```python
from build123d import *
from build123d.topology import SkipClean

# Parameters (mm, degrees)
SKETCH_1_R               = 705
EXTRUDE_1_DEPTH          = 25
CUT_EXTRUDE_1_REACH      = 999.334
PATTERN_CIRCULAR_1_COUNT = 4
CUT_EXTRUDE_2_REACH      = 999.177
SKETCH_8_R               = 60
CUT_EXTRUDE_3_DEPTH      = 998.177266087
CUT_EXTRUDE_7_DEPTH      = 998.177266087
CUT_EXTRUDE_8_DEPTH      = 998.177266087
SKETCH_18_R              = 40
CUT_EXTRUDE_13_DEPTH     = 998.177266087
SKETCH_19_R              = 3
CUT_EXTRUDE_14_DEPTH     = 100
CUT_EXTRUDE_15_DEPTH     = 8


with BuildPart() as part:
    # 草图1 → 凸台-拉伸1 (new body)
    with BuildSketch(Plane(origin=(0, 0, 0), x_dir=(1, 0, 0), z_dir=(0, 1, 0))):
        with Locations(Location((0, 0, 0), (0, 0, 270))):
            Circle(SKETCH_1_R)
    extrude(amount=EXTRUDE_1_DEPTH)

    # 草图2 → 切除-拉伸1 (cut, up to next)
    with BuildSketch(Plane(origin=(0, 25, 0), x_dir=(1, 0, 0), z_dir=(0, 1, 0)), mode=Mode.PRIVATE) as cut_extrude_1_sk1:
        with BuildLine():
            Line((-12.5, -699.994189271), (-12.5, -704.889175687))
            ThreePointArc((-12.5, -704.889175687), (0, -705), (12.5, -704.889175687))
            Line((12.5, -704.889175687), (12.5, -699.994189271))
            Line((12.5, -699.994189271), (0, -678.343554177))
            Line((0, -678.343554177), (-12.5, -699.994189271))
        make_face()
    cut_extrude_1_tool1 = extrude(cut_extrude_1_sk1.sketch, amount=-CUT_EXTRUDE_1_REACH, mode=Mode.PRIVATE) & part.part
    cut_extrude_1 = cut_extrude_1_tool1.solids().sort_by_distance((0, 25, 695.82939))[0]
    add(cut_extrude_1, mode=Mode.SUBTRACT)

    # 阵列(圆周)1: 切除-拉伸1 ×4 about axis
    pattern_circular_1_axis = Axis((0, 0, 0), (0, 1, 0))
    for i in range(1, PATTERN_CIRCULAR_1_COUNT):
        add(cut_extrude_1.rotate(pattern_circular_1_axis, i * 360 / PATTERN_CIRCULAR_1_COUNT), mode=Mode.SUBTRACT)

    # 草图8 → 切除-拉伸2 (cut, up to next)
    with BuildSketch(Plane(origin=(0, 25, 0), x_dir=(1, 0, 0), z_dir=(0, 1, 0)), mode=Mode.PRIVATE) as cut_extrude_2_sk1:
        with Locations(Location((247.487373415, -247.487373415, 0), (0, 0, 270))):
            Circle(SKETCH_8_R)
    cut_extrude_2_tool1 = extrude(cut_extrude_2_sk1.sketch, amount=-CUT_EXTRUDE_2_REACH, mode=Mode.PRIVATE) & part.part
    # 草图8 → 切除-拉伸2 (cut, up to next)
    with BuildSketch(Plane(origin=(0, 25, 0), x_dir=(1, 0, 0), z_dir=(0, 1, 0)), mode=Mode.PRIVATE) as cut_extrude_2_sk2:
        with Locations(Location((-212.132034356, -212.132034356, 0), (0, 0, 270))):
            Circle(SKETCH_8_R)
    cut_extrude_2_tool2 = extrude(cut_extrude_2_sk2.sketch, amount=-CUT_EXTRUDE_2_REACH, mode=Mode.PRIVATE) & part.part
    # 草图8 → 切除-拉伸2 (cut, up to next)
    with BuildSketch(Plane(origin=(0, 25, 0), x_dir=(1, 0, 0), z_dir=(0, 1, 0)), mode=Mode.PRIVATE) as cut_extrude_2_sk3:
        with Locations(Location((-212.132034356, 212.132034356, 0), (0, 0, 270))):
            Circle(SKETCH_8_R)
    cut_extrude_2_tool3 = extrude(cut_extrude_2_sk3.sketch, amount=-CUT_EXTRUDE_2_REACH, mode=Mode.PRIVATE) & part.part
    # 草图8 → 切除-拉伸2 (cut, up to next)
    with BuildSketch(Plane(origin=(0, 25, 0), x_dir=(1, 0, 0), z_dir=(0, 1, 0)), mode=Mode.PRIVATE) as cut_extrude_2_sk4:
        with Locations(Location((212.132034356, 212.132034356, 0), (0, 0, 270))):
            Circle(SKETCH_8_R)
    cut_extrude_2_tool4 = extrude(cut_extrude_2_sk4.sketch, amount=-CUT_EXTRUDE_2_REACH, mode=Mode.PRIVATE) & part.part
    add(cut_extrude_2_tool1.solids().sort_by_distance((247.487373, 25, 247.487373))[0], mode=Mode.SUBTRACT)
    add(cut_extrude_2_tool2.solids().sort_by_distance((-212.132034, 25, 212.132034))[0], mode=Mode.SUBTRACT)
    add(cut_extrude_2_tool3.solids().sort_by_distance((-212.132034, 25, -212.132034))[0], mode=Mode.SUBTRACT)
    add(cut_extrude_2_tool4.solids().sort_by_distance((212.132034, 25, -212.132034))[0], mode=Mode.SUBTRACT)

    # 草图9 → 切除-拉伸3 (cut, through all)
    with BuildSketch(Plane(origin=(0, 25, 0), x_dir=(1, 0, 0), z_dir=(0, 1, 0))):
        Polygon((388.545974556, -190.514916099), (515.825974556, -63.236474876), (643.105974556, -190.514916099), (515.825974556, -317.793357321), align=None)
    extrude(amount=-CUT_EXTRUDE_3_DEPTH, mode=Mode.SUBTRACT)

    # 草图13 → 切除-拉伸7 (cut, through all)
    with BuildSketch(Plane.XZ):
        Polygon((165.039343844, 165.039343844), (398.093317994, -68.014630305), (332.597815836, -133.510132463), (99.543841687, 99.543841687), align=None)
    extrude(amount=-CUT_EXTRUDE_7_DEPTH, mode=Mode.SUBTRACT)

    # 草图14 → 切除-拉伸8 (cut, through all)
    with BuildSketch(Plane.XZ):
        Polygon((165.039343844, 165.039343844), (99.543841687, 99.543841687), (76.501917102, 122.585766271), (141.99741926, 188.081268429), align=None)
    extrude(amount=-CUT_EXTRUDE_8_DEPTH, mode=Mode.SUBTRACT)

    # 草图18 → 切除-拉伸13 (cut, through all)
    with BuildSketch(Plane(origin=(0, 25, 0), x_dir=(1, 0, 0), z_dir=(0, 1, 0))):
        with Locations(Location((-156.54417142, -331.667653242, 0), (0, 0, 270))):
            Circle(SKETCH_18_R)
    extrude(amount=-CUT_EXTRUDE_13_DEPTH, mode=Mode.SUBTRACT)

    # 草图19 → 切除-拉伸14 (cut)
    with BuildSketch(Plane.XZ):
        with Locations(Location((-10.777149233, 258.231573261, 0), (0, 0, 270))):
            Circle(SKETCH_19_R)
        with Locations(Location((-191.089378436, 438.543802464, 0), (0, 0, 270))):
            Circle(SKETCH_19_R)
        with Locations(Location((3.36498639, 272.373708885, 0), (0, 0, 90))):
            Circle(SKETCH_19_R)
        with Locations(Location((-176.947242812, 452.685938088, 0), (0, 0, 90))):
            Circle(SKETCH_19_R)
    extrude(amount=-CUT_EXTRUDE_14_DEPTH, mode=Mode.SUBTRACT)

    # 草图20 → 切除-拉伸15 (cut)
    with SkipClean():  # the faces are left unmerged after this step: merging them gives an invalid solid
        with BuildSketch(Plane(origin=(0, 25, 0), x_dir=(1, 0, 0), z_dir=(0, 1, 0))):
            with BuildLine():
                Line((169.705627485, 169.705627485), (84.852813742, 254.558441227))
                ThreePointArc((84.852813742, 254.558441227), (84.852813742, 339.41125497), (169.705627485, 339.41125497))
                Line((169.705627485, 339.41125497), (254.558441227, 254.558441227))
                ThreePointArc((254.558441227, 254.558441227), (254.558441227, 169.705627485), (169.705627485, 169.705627485))
            make_face()
            with BuildLine():
                Line((-169.705627485, -169.705627485), (-254.558441227, -84.852813742))
                ThreePointArc((-254.558441227, -84.852813742), (-339.41125497, -84.852813742), (-339.41125497, -169.705627485))
                Line((-339.41125497, -169.705627485), (-254.558441227, -254.558441227))
                ThreePointArc((-254.558441227, -254.558441227), (-169.705627485, -254.558441227), (-169.705627485, -169.705627485))
            make_face()
            with BuildLine():
                Line((-169.705627485, 169.705627485), (-254.558441227, 84.852813742))
                ThreePointArc((-254.558441227, 84.852813742), (-339.41125497, 84.852813742), (-339.41125497, 169.705627485))
                Line((-339.41125497, 169.705627485), (-254.558441227, 254.558441227))
                ThreePointArc((-254.558441227, 254.558441227), (-169.705627485, 254.558441227), (-169.705627485, 169.705627485))
            make_face()
            with BuildLine():
                Line((289.913780286, -289.913780286), (205.060966544, -374.766594029))
                ThreePointArc((205.060966544, -374.766594029), (120.208152802, -374.766594029), (120.208152802, -289.913780286))
                Line((120.208152802, -289.913780286), (205.060966544, -205.060966544))
                ThreePointArc((205.060966544, -205.060966544), (289.913780286, -205.060966544), (289.913780286, -289.913780286))
            make_face()
        extrude(amount=-CUT_EXTRUDE_15_DEPTH, mode=Mode.SUBTRACT)


solid = part.part
```
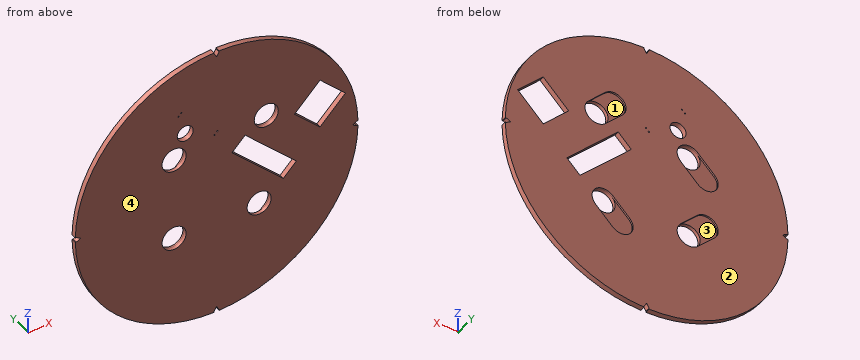
The listing builds one solid part. Answer for the finished solid, in the listing's coordinates (mm). Face numbers are marked on the shaded views. A direction names the side the tool comes from. Give positions to 0.01 mm unless a question says otherwise; leave off trailing zeros. Loops run counter-clockwise (first coordinate to the right, second up) from the corner with the lowest first, then second, coordinate; pieces in that order, holes last. Notation, with made-up numbers: (45, 39.5) - (88, 39.5) arc R3 cw to (88, 44.5) - close; hole circle Ø6 at (22.25, 25). An arc over 180 degrees is marked (long way). Return JSON: item names as keys, results as strings. Group by question number.
1. Find section C-C (y = 13.25). State how many separate pieces and enclosed holes the cut face has, then the cut area to 3 significant figures.
2. Determine the mould class of the marked faces 1 and 2 for opening direction X: pulls with the +X half, pulls with the -X half, needs draft (parallel to the pull), parting line crosses it, or undercut.
3. Find section A-A (x = 571.5). Write down the section's boundary in (y, z).
4. Find section B-B (z = -471). Write down the section's boundary in (x, y).
5. Which of the six approach directions +Z, -Z, +X, -X, +Y, -Y give full straight-line access (tool end or side, diameter ignored) to the marked faces 3 and 4?
6. Find section D-D (x = -490). Write down the section's boundary in (y, z).
7. Straight lines are drawn through the part: line 1 (Z direction, x = 257.5, y = 15.75); line 2 (Z direction, x = 234.5, y = 23.75); line 3 (X direction, y = 3, z = 144). For each, find the intervals that lie inside material, in ascending order. Write a range as [from, to].
8. Given pin 1 Ø3 at (x, y) = (427.5, 18.5) entering from +Z; pin 2 Ø12 at (y, z) = (10, 110.5) entering from -X; pin 3 Ø5 at (x, y) = (-358.5, 17.5) entering from -Z, each flat-ended and moving along its own axis, determine where each tip first touches the part or whether it passes through.
Verdict:
{
 "1": {"separate pieces": "1", "enclosed holes": "11", "area": "1,440,000 mm^2"},
 "2": {"face 1": "undercut", "face 2": "needs draft"},
 "3": {"outline": "(0, -412.81) - (25, -412.81) - (25, 118.91) - (0, 118.91) - close; (0, 262.12) - (25, 262.12) - (25, 412.81) - (0, 412.81) - close"},
 "4": {"outline": "(-524.58, 0) - (524.58, 0) - (524.58, 25) - (-524.58, 25) - close"},
 "5": {"face 3": "+Y", "face 4": "+Z, -Z, +X, -X, -Y"},
 "6": {"outline": "(0, -506.88) - (25, -506.88) - (25, 506.88) - (0, 506.88) - close"},
 "7": {"line 1": "z = [-656.29, -251.4], [-172.87, -58.41], [72.58, 188.33], [306.65, 656.29]", "line 2": "z = [-664.86, -274.62], [-156.46, -35.41], [95.58, 188.91], [345.33, 664.86]", "line 3": "x = [-690.14, 97.92], [186.08, 435.06], [596.59, 690.14]"},
 "8": {"pin 1": "stops at z = 561.74", "pin 2": "stops at x = -697.21", "pin 3": "stops at z = -608.51"}
}
